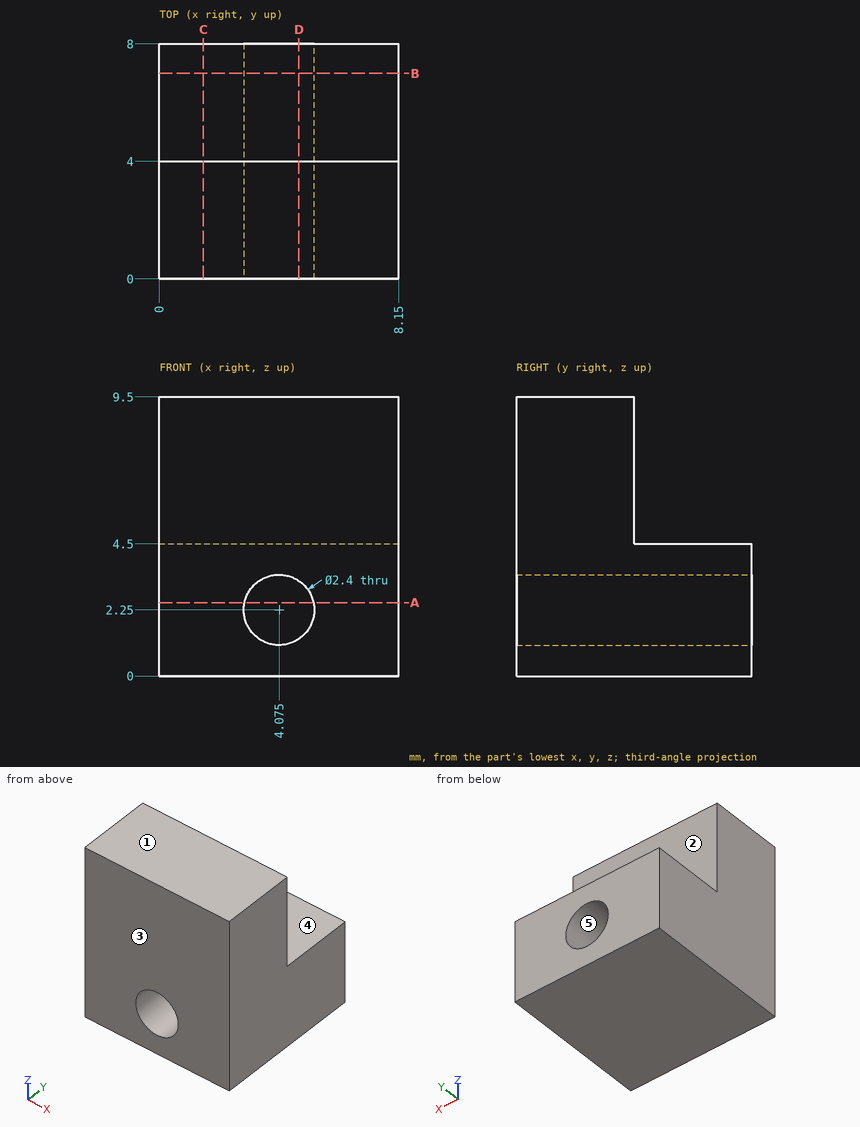
Job drawing, mm, ordinate dimensions from the low corner. One solid piece. A direction names the side the tool comes from. Coordinates: 2 decimals unless noted, no trailing zeros. Loops run counter-clockwise (first coordinate to the right, second up) from the corner with the lowest first, then second, coordinate; pieces in that order, holes last. Notation, with made-up numbers: (4.25, 36) - (18.25, 36) arc R18 ccw to (18.25, 42) - close; hole circle Ø8 at (25.5, -5). An arc over 180 degrees is marked (long way). Write item = value, one per line. Start each with the question number.
Q1. Cut at A-A, the plane z = 2.5. List the corners of the cut face in (x, y), then the cut area to 3 significant figures.
Q2. Cut at C-C, the plane x = 1.5. List the corners of the cut face in (y, z), then the cut area to 3 significant figures.
Q3. Flat gauge pins, fed straight in: pin 1 Ø1.5 at (x, y) = (1, 1.5) entering from -Z; pin 2 Ø3 at (x, z) = (6, 7.5) entering from +Y; pin 3 Ø2 at (x, z) = (4.075, 2.25) entering from -Y. Where does each tip first touch, or does it go through?
Q4. Cut at B-B, the plane y = 7. List the corners of the cut face in (x, z) (3 decimals).
Q5. Drill centre lines: L1, parallel to Y at x = 2.5, z = 9; L2, parallel to Z at x = 3, y = 3.75; L3, parallel to Z at x = 4, y = 1. Where is each one in solid material? Low to high.
Q6. Cut at D-D, the plane x = 4.75. List the corners of the cut face in (y, z).
Q7. Which spindle directions (+Z, -Z, +X, -X, +Y, -Y) get a long thin tool onto all of the face, cutting with end or side? Do the marked faces 1 and 2. Say none if no direction does.
Q8. Pull direction Z, two halves, no side cores. Call the marked faces 3, 4 and 5: pulls with the +Z half, pulls with the -Z half, needs draft (parallel to the pull), parting line crosses it, or undercut.
Computed:
q1.outline = (0, 0) - (2.9, 0) - (2.9, 8) - (0, 8) - close; (5.25, 0) - (8.15, 0) - (8.15, 8) - (5.25, 8) - close
q1.area = 46.4 mm²
q2.outline = (0, 0) - (8, 0) - (8, 4.5) - (4, 4.5) - (4, 9.5) - (0, 9.5) - close
q2.area = 56.0 mm²
q3.pin_1 = 0
q3.pin_2 = 4
q3.pin_3 = through
q4.outline = (0, 0) - (8.15, 0) - (8.15, 4.5) - (0, 4.5) - close; hole circle Ø2.4 at (4.075, 2.25)
q5.L1 = 0 to 4
q5.L2 = 0 to 1.72, 2.78 to 9.5
q5.L3 = 0 to 1.05, 3.45 to 9.5
q6.outline = (0, 0) - (8, 0) - (8, 1.26) - (0, 1.26) - close; (0, 3.24) - (8, 3.24) - (8, 4.5) - (4, 4.5) - (4, 9.5) - (0, 9.5) - close
q7.face_1 = +Z, +X, -X, +Y, -Y
q7.face_2 = +Z, +X, -X, +Y
q8.face_3 = needs draft
q8.face_4 = pulls with the +Z half
q8.face_5 = undercut
